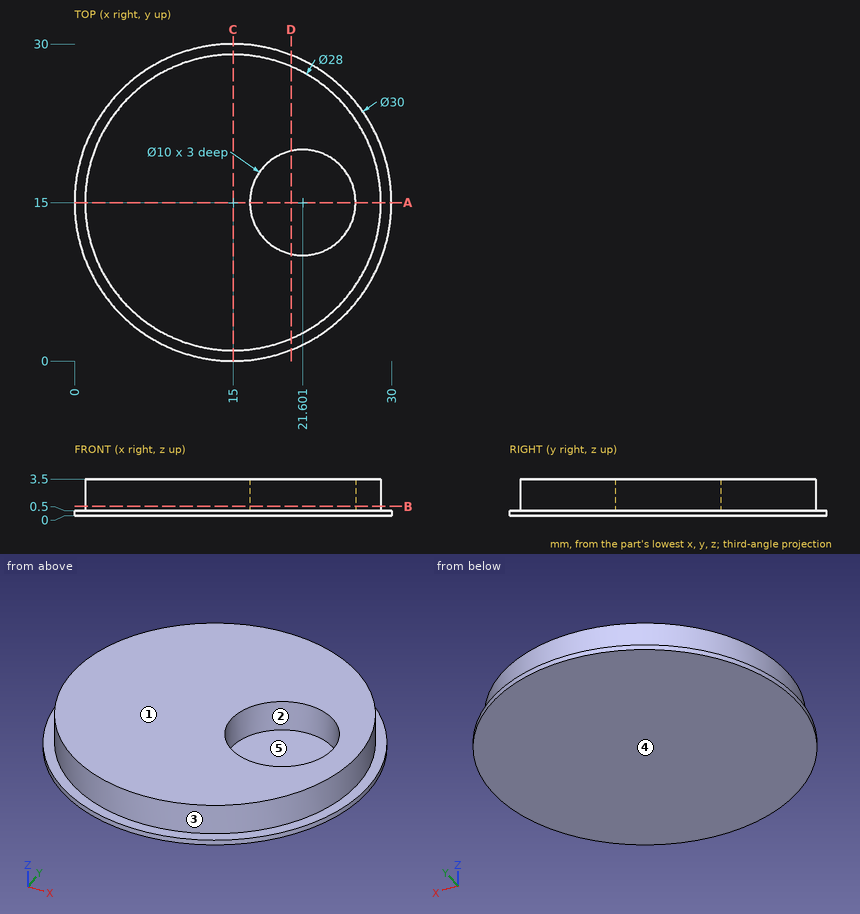
Job drawing, mm, ordinate dimensions from the low corner. One solid piece. A direction names the side the tool comes from. Coordinates: 2 decimals unless noted, no trailing zeros. Loops run counter-clockwise (first coordinate to the right, second up) from the corner with the lowest first, then second, coordinate; pieces in that order, holes last. Notation, with made-up numbers: (70.25, 61) - (103.25, 61) arc R24 ccw to (103.25, 86) - close; hole circle Ø10 at (-12.5, 54). An arc over 180 degrees is marked (long way). Answer as a JSON object with one key per item and string values. Group by question number.
(1) Cut at D-D (x = 20.5). Give the cut face in (y, z) (1 decimal).
(2) Cut at B-B (z = 0.9). Give the cut face in (x, y), then the cut area to 3 significant figures.
(3) Cut at C-C (x = 15). Give the cut face in (y, z).
(4) Two-plate mould, pull along Y, no slides. Class the marked faces 3, 4 and 5: released by +Y, released by -Y, zero draft, split by the parting line, or undercut.
(5) Tool access for the marked faces 1 and 2: list every direction of +Z, -Z, +X, -X, +Y, -Y with a clear straight run to the whole face (end or side of a thin tool).
(6) Cut at A-A (y = 15). Give the cut face in (x, z).
(7) Flat gauge pins, fed straight in: pin 1 (4 mm diameter, centred on x = 19, y = 10, fed in from -Z); pin 2 (1 mm diameter, centred on y = 4.5, z = 2, fed in from +X); pin 3 (6 mm diameter, centred on x = 21.6, y = 15, fed in from +Z); pin 4 (1 mm diameter, centred on x = 27, z = 1.5, fed in from -Y) (1 decimal). Where does each tip first touch, or does it go through?
(8) Probe line 1 along Z through (x, y) = (25.5, 17.5); line 2 along Y through (x, z) = (18.25, 1.1); line 3 along Y through (x, z) = (23, 2.05). List the from-to ranges inside material, lowest first.
Geometry says:
{
 "1": {"outline": "(1, 0) - (29, 0) - (29, 0.5) - (27.9, 0.5) - (27.9, 3.5) - (19.9, 3.5) - (19.9, 0.5) - (10.1, 0.5) - (10.1, 3.5) - (2.1, 3.5) - (2.1, 0.5) - (1, 0.5) - close"},
 "2": {"outline": "circle Ø28 at (15, 15); hole circle Ø10 at (21.6, 15)", "area": "537 mm^2"},
 "3": {"outline": "(0, 0) - (30, 0) - (30, 0.5) - (29, 0.5) - (29, 3.5) - (1, 3.5) - (1, 0.5) - (0, 0.5) - close"},
 "4": {"face 3": "split by the parting line", "face 4": "zero draft", "face 5": "undercut"},
 "5": {"face 1": "+Z, +X, -X, +Y, -Y", "face 2": "+Z"},
 "6": {"outline": "(0, 0) - (30, 0) - (30, 0.5) - (29, 0.5) - (29, 3.5) - (26.6, 3.5) - (26.6, 0.5) - (16.6, 0.5) - (16.6, 3.5) - (1, 3.5) - (1, 0.5) - (0, 0.5) - close"},
 "7": {"pin 1": "stops at z = 0", "pin 2": "stops at x = 24.8", "pin 3": "stops at z = 0.5", "pin 4": "stops at y = 7"},
 "8": {"line 1": "z = 0 to 0.5", "line 2": "y = 1.38 to 11.29, 18.71 to 28.62", "line 3": "y = 3.51 to 10.2, 19.8 to 26.49"}
}
